```python
from build123d import *

# Parameters (mm, degrees)
SKETCH1_W               = 150
SKETCH1_H               = 120
BOSS_EXTRUDE1_DEPTH     = 10
SKETCH2_R               = 4
CUT_EXTRUDE1_DEPTH      = 30
CROQUIS4_R              = 2.5
SALIENTE_EXTRUIR2_DEPTH = 10
CROQUIS5_R              = 1.75
CORTAR_EXTRUIR1_DEPTH   = 9
CROQUIS6_W              = 150
CROQUIS6_H              = 100
SALIENTE_EXTRUIR3_DEPTH = 10
CROQUIS9_W              = 150
CROQUIS9_H              = 100
SALIENTE_EXTRUIR4_DEPTH = 10
CROQUIS10_R             = 4
CORTAR_EXTRUIR2_DEPTH   = 30
FILLET1_R               = 8


with BuildPart() as part:
    # Sketch1 → Boss-Extrude1 (new body)
    with BuildSketch(Plane.XY):
        with Locations((75, 0)):
            Rectangle(SKETCH1_W, SKETCH1_H)
    extrude(amount=BOSS_EXTRUDE1_DEPTH)

    # Sketch2 → Cut-Extrude1 (cut)
    with BuildSketch(Plane.ZY):
        with Locations((5, 0)):
            Circle(SKETCH2_R)
        with Locations((5, 30)):
            Circle(SKETCH2_R)
        with Locations((5, -30)):
            Circle(SKETCH2_R)
    extrude(amount=-CUT_EXTRUDE1_DEPTH, mode=Mode.SUBTRACT)

    # Croquis4 → Saliente-Extruir2 (add)
    with BuildSketch(Plane.XY.offset(10)):
        with Locations((47.900115216, 0.5)):
            Circle(CROQUIS4_R)
        with Locations((105.9, 0.615607451)):
            Circle(CROQUIS4_R)
        with Locations((105.9, -48.5)):
            Circle(CROQUIS4_R)
        with Locations((47.900115216, -48.5)):
            Circle(CROQUIS4_R)
    extrude(amount=SALIENTE_EXTRUIR2_DEPTH)

    # Croquis5 → Cortar-Extruir1 (cut)
    with BuildSketch(Plane.XY.offset(20)):
        with Locations((47.900115216, 0.5)):
            Circle(CROQUIS5_R)
        with Locations((47.900115216, -48.5)):
            Circle(CROQUIS5_R)
        with Locations((105.9, -48.5)):
            Circle(CROQUIS5_R)
        with Locations((105.9, 0.615607451)):
            Circle(CROQUIS5_R)
    extrude(amount=-CORTAR_EXTRUIR1_DEPTH, mode=Mode.SUBTRACT)

    # Croquis6 → Saliente-Extruir3 (add)
    with BuildSketch(Plane.XZ.offset(60)):
        with Locations((75, 50)):
            Rectangle(CROQUIS6_W, CROQUIS6_H)
    extrude(amount=SALIENTE_EXTRUIR3_DEPTH)

    # Croquis9 → Saliente-Extruir4 (add)
    with BuildSketch(Plane(origin=(0, 60, 0), x_dir=(1, 0, 0), z_dir=(0, 1, 0))):
        with Locations((75, -50)):
            Rectangle(CROQUIS9_W, CROQUIS9_H)
    extrude(amount=SALIENTE_EXTRUIR4_DEPTH)

    # Croquis10 → Cortar-Extruir2 (cut)
    with BuildSketch(Plane(origin=(150, 0, 0), x_dir=(0, 0, -1), z_dir=(1, 0, 0))):
        with Locations((-81.62673219, 65)):
            Circle(CROQUIS10_R)
        with Locations((-41.62673219, 65)):
            Circle(CROQUIS10_R)
        with Locations((-81.62673219, -65)):
            Circle(CROQUIS10_R)
        with Locations((-41.62673219, -65)):
            Circle(CROQUIS10_R)
    extrude(amount=-CORTAR_EXTRUIR2_DEPTH, mode=Mode.SUBTRACT)

    # Fillet1
    fillet1_edges = [part.edges().sort_by_distance(p)[0] for p in [
        (75, -70, 0),
        (75, 70, 0),
    ]]
    fillet(fillet1_edges, radius=FILLET1_R)


solid = part.part
```
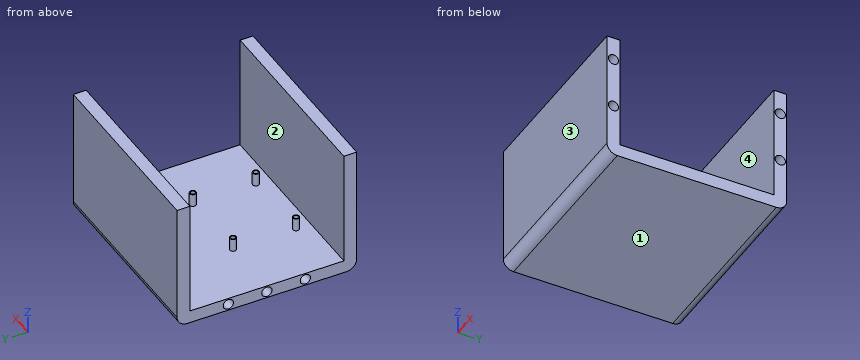
CAD build for the part. Positions are in the model's coordinates, mm. Face numbers are marked on the shaded views. Give positions to 0.01 mm unless a question says otherwise; leave off trailing zeros. Order: outer loops, then holes, each group sorted by start corner. A loop starts at its lowest first (then second) coordinate and runs counter-clockwise, first axis right, second up. Notation, with made-up numbers: M 49,-24 L 72,-24 A22 ccw 72,-10 Z; hole C 72.5,74.25 d5. An arc over 180 degrees is marked long. Put each result on its own line as item: value. Start each with the question number.
(1) Saw through at C-C, the plane z = 13. Give the number of separate pieces and of enclosed holes in the cut face, then the cut area to 3 significant figures.
(2) Drill centre lines: line 1 along Y through (x, z) = (105.9, 17.5); line 2 along Y through (x, z) = (82, 68.5); line 3 along Y through (x, z) = (138, 40). Where is each one in solid material? Low to high.
(3) Saw through at A-A, the plane z = 90. Write the cut outline in (x, y).
(4) Mould opens along Y. For the marked faces 1, 2, 3 and 4 say: +Y half, -Y half, draft (parallel to the pull), parting line (faces both ways), or undercut.
(5) Flat gauge pins, fed straight in: pin 1 Ø2.5 at (x, y) = (47, 0) entering from +Z; pin 2 Ø2 at (x, y) = (97.5, 42.5) entering from +Z; pin 3 Ø2.5 at (y, z) = (-64, 81.5) entering from +X. Where does each tip first touch, or does it go through?
(6) Saw through at B-B, the plane x = 138.5. Write the cut outline in (y, z), then the cut area to 3 significant figures.
(7) Saw through at D-D, the plane y = 30. Write the cut outline in (x, z), then the cut area to 3 significant figures.
Check result:
1. separate pieces: 6
1. enclosed holes: 4
1. area: 3,040 mm2
2. line 1: y = -70 to -60, -51 to -50.25, -46.75 to -46, -1.88 to -1.13, 2.37 to 3.12, 60 to 70
2. line 2: y = -70 to -60, 60 to 70
2. line 3: y = -70 to -68.65, -61.35 to -60, 60 to 61.35, 68.65 to 70
3. outline: M 0,-70 L 150,-70 L 150,-60 L 0,-60 Z; M 0,60 L 150,60 L 150,70 L 0,70 Z
4. face 1: draft
4. face 2: undercut
4. face 3: -Y half
4. face 4: undercut
5. pin 1: stops at z = 20
5. pin 2: stops at z = 10
5. pin 3: stops at x = 120
6. outline: M -70,8 A8 ccw -62,0 L 62,0 A8 ccw 70,8 L 70,100 L 60,100 L 60,10 L -60,10 L -60,100 L -70,100 Z; hole C -65,41.63 d8; hole C -65,81.63 d8; hole C 65,41.63 d8; hole C 65,81.63 d8
6. area: 2,970 mm2
7. outline: M 0,0 L 150,0 L 150,10 L 0,10 L 0,9 L 30,9 L 30,1 L 0,1 Z
7. area: 1,260 mm2
